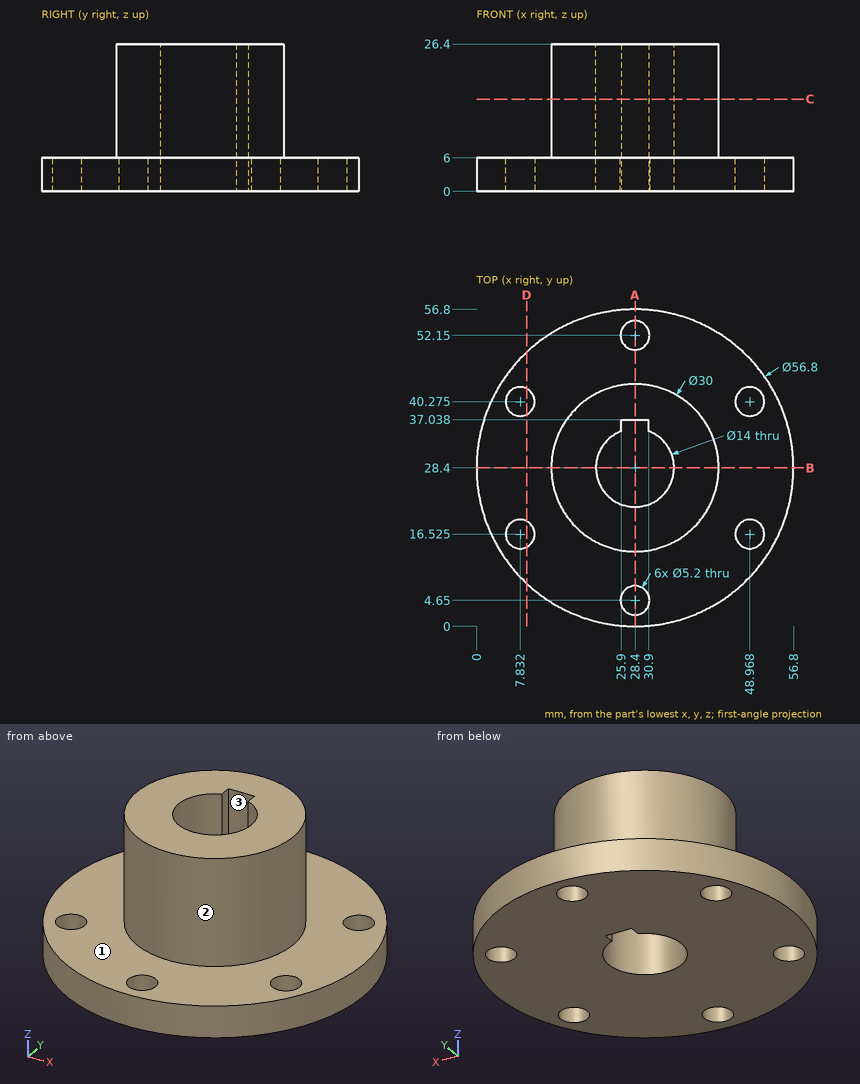
Print and shaded views of the part. All mm, measured from the part's lowest x, y and z. Round coordinates to 2 decimals unless told otherwise and drop trailing zeros. Order: outer loops, then holes, each group sorted by start corner. A loop starts at its lowest first (then second) coordinate and runs counter-clockwise, first axis right, second up. Notation, with made-up numbers: (24.25, 72) - (52.25, 72) arc R20 cw to (52.25, 90) - close; hole circle Ø7 at (85.25, 36). An arc over 180 degrees is marked (long way). Use a Markdown table: item, result.
1) Saw through at B-B on y = 28.4. Write the cut outline in (x, z), and give its area (3 significant figures).
Recorded:
| item | result |
|---|---|
| outline | (0, 0) - (21.4, 0) - (21.4, 26.4) - (13.4, 26.4) - (13.4, 6) - (0, 6) - close; (35.4, 0) - (56.8, 0) - (56.8, 6) - (43.4, 6) - (43.4, 26.4) - (35.4, 26.4) - close |
| area | 583 mm² |
2) Flat gauge pins, fed straight in: pin 1 Ø4 at (x, z) = (19, 5.5) entering from -Y; pin 2 Ø4 at (x, y) = (7.83, 40.28) entering from +Z; pin 3 Ø1.7 at (y, z) = (36, 8) entering from +X (1 decimal); pin 4 Ø3 at (x, y) = (23, 10.5) entering from +Z. Where does each tip first touch, or does it go through?
Recorded:
| item | result |
|---|---|
| pin 1 | stops at y = 0.98 |
| pin 2 | passes through |
| pin 3 | stops at x = 41.8 |
| pin 4 | stops at z = 6 |
3) Pull direction Y, two halves, no side cores. Call the marked faces 1, 2 and 3: pulls with the +Y half, pulls with the -Y half, needs draft (parallel to the pull), parting line crosses it, or undercut.
Recorded:
| item | result |
|---|---|
| face 1 | needs draft |
| face 2 | parting line crosses it |
| face 3 | undercut |
4) Wall check: L1, parallel to Y at x = 28.4, z = 1.7; L2, parallel to X at y = 28, z = 19 (1 decimal); L3, parallel to Z at x = 20.5, y = 11. Give the ranges that are in metal, low to high.
Recorded:
| item | result |
|---|---|
| L1 | y = 0 to 2.05, 7.25 to 21.4, 37.04 to 49.55, 54.75 to 56.8 |
| L2 | x = 13.4 to 21.4, 35.4 to 43.4 |
| L3 | z = 0 to 6 |
5) Saw through at A-A on x = 28.4. Write the cut outline in (y, z).
Recorded:
| item | result |
|---|---|
| outline | (0, 0) - (2.05, 0) - (2.05, 6) - (0, 6) - close; (7.25, 0) - (21.4, 0) - (21.4, 26.4) - (13.4, 26.4) - (13.4, 6) - (7.25, 6) - close; (37.04, 0) - (49.55, 0) - (49.55, 6) - (43.4, 6) - (43.4, 26.4) - (37.04, 26.4) - close; (54.75, 0) - (56.8, 0) - (56.8, 6) - (54.75, 6) - close |
6) Saw through at C-C on z = 16.5. Write the cut outline in (x, y), and give its area (3 significant figures).
Recorded:
| item | result |
|---|---|
| outline | circle Ø30 at (28.4, 28.4); hole (25.9, 34.94) arc R7 ccw (long way) to (30.9, 34.94) - (30.9, 37.04) - (25.9, 37.04) - close |
| area | 544 mm² |
7) Saw through at D-D on x = 9. Write the cut outline in (y, z).
Recorded:
| item | result |
|---|---|
| outline | (7.66, 0) - (14.2, 0) - (14.2, 6) - (7.66, 6) - close; (18.85, 0) - (37.95, 0) - (37.95, 6) - (18.85, 6) - close; (42.6, 0) - (49.14, 0) - (49.14, 6) - (42.6, 6) - close |
